Check sheet for the modelled part. Datum: model origin and axes. Units: mm. Give positions to 0.01 mm unless a question says otherwise; leave off trailing zeros. Loops run counter-clockwise (first coordinate to the right, second up) from the corner with the lowest first, then second, coordinate; pieces in that order, holes last. Notation, with made-up numbers: (87, 17) -> (97, 17) arc R24 ccw to (97, 37) -> close; hole circle Ø6 at (60.25, -39). An arc over 180 degrees is marked (long way). Answer as CSV lines item,"result". Start each with the question number.
(1) Section check A-A on y = 0. Enter the section's corners in (x, z) (3 decimals), plus the area to 3 significant figures.
(2) Release check for a two-part mould opening along X. For faces 1 (the face through (-42.5, -1, 4)), 2 (the face through (-1, 42.5, 4)), 3 (the face through (20.065, 23.774, 4.338)), 4 (the face through (42.5, -1, 4)) record: pulls with the +X half, pulls with the -X half, needs draft (parallel to the pull), parting line crosses it, or undercut.
(3) Section check C-C on z = 5.5. Enter the section's corners in (x, y) (3 decimals), plus the area to 3 significant figures.
(4) Section check D-D on y = 22. Enter the section's corners in (x, z) (3 decimals), plus the area to 3 significant figures.
(5) Material ranges on line 1 (Y direction, x = -22, z = 4.5) (3 decimals); line 2 (Y direction, x = 0, z = 6.25) (3 decimals); line 3 (X direction, y = 1.5, z = 8), recorded low to high. Write a range as from..to.
from build123d import *

# Parameters (mm, degrees)
SKETCH_W  = 85
SKETCH_H  = 85
SKETCH_R  = 2.625
PAD_DEPTH = 8.8


with BuildPart() as part:
    # Sketch → Pad (new body)
    with BuildSketch(Plane.XY):
        Rectangle(SKETCH_W, SKETCH_H)
        with Locations((-22, 22)):
            Circle(SKETCH_R, mode=Mode.SUBTRACT)
        with Locations((-22, 0)):
            Circle(SKETCH_R, mode=Mode.SUBTRACT)
        with Locations((-22, -22)):
            Circle(SKETCH_R, mode=Mode.SUBTRACT)
        Circle(SKETCH_R, mode=Mode.SUBTRACT)
        with Locations((22, 22)):
            Circle(SKETCH_R, mode=Mode.SUBTRACT)
        with Locations((22, 0)):
            Circle(SKETCH_R, mode=Mode.SUBTRACT)
        with Locations((22, -22)):
            Circle(SKETCH_R, mode=Mode.SUBTRACT)
    extrude(amount=PAD_DEPTH)


solid = part.part
Working result:
1,outline,"(-42.5, 0) -> (-24.625, 0) -> (-24.625, 8.8) -> (-42.5, 8.8) -> close; (-19.375, 0) -> (-2.625, 0) -> (-2.625, 8.8) -> (-19.375, 8.8) -> close; (2.625, 0) -> (19.375, 0) -> (19.375, 8.8) -> (2.625, 8.8) -> close; (24.625, 0) -> (42.5, 0) -> (42.5, 8.8) -> (24.625, 8.8) -> close"
1,area,"609 mm^2"
2,face 1,"pulls with the -X half"
2,face 2,"needs draft"
2,face 3,"undercut"
2,face 4,"pulls with the +X half"
3,outline,"(-42.5, -42.5) -> (42.5, -42.5) -> (42.5, 42.5) -> (-42.5, 42.5) -> close; hole circle Ø5.25 at (-22, -22); hole circle Ø5.25 at (-22, 0); hole circle Ø5.25 at (-22, 22); hole circle Ø5.25 at (0, 0); hole circle Ø5.25 at (22, -22); hole circle Ø5.25 at (22, 0); hole circle Ø5.25 at (22, 22)"
3,area,"7,070 mm^2"
4,outline,"(-42.5, 0) -> (-24.625, 0) -> (-24.625, 8.8) -> (-42.5, 8.8) -> close; (-19.375, 0) -> (19.375, 0) -> (19.375, 8.8) -> (-19.375, 8.8) -> close; (24.625, 0) -> (42.5, 0) -> (42.5, 8.8) -> (24.625, 8.8) -> close"
4,area,"656 mm^2"
5,line 1,"y = -42.5..-24.625, -19.375..-2.625, 2.625..19.375, 24.625..42.5"
5,line 2,"y = -42.5..-2.625, 2.625..42.5"
5,line 3,"x = -42.5..-24.15, -19.85..-2.15, 2.15..19.85, 24.15..42.5"
